```python
from build123d import *

# Parameters (mm, degrees)
SKETCH1_R           = 1.5
BOSS_EXTRUDE1_DEPTH = 2
SKETCH2_R           = 1.5
CUT_EXTRUDE1_DEPTH  = 55
FILLET1_R           = 1


with BuildPart() as part:
    # Sketch1 → Boss-Extrude1 (new body)
    with BuildSketch(Plane(origin=(0, 0, 0), x_dir=(1, 0, 0), z_dir=(0, 1, 0))):
        Polygon((0, 5), (0, -5), (3, -5), (3, 0), (8.68728571, 0), (8.68728571, -5), (11.68728571, -5), (11.68728571, 0), (38.51271429, 0), (38.51271429, -5), (41.51271429, -5), (41.51271429, 0), (47.2, 0), (47.2, -5), (50.2, -5), (50.2, 5), align=None)
        with Locations((2.5, 2.5)):
            Circle(SKETCH1_R, mode=Mode.SUBTRACT)
        with Locations((47.7, 2.5)):
            Circle(SKETCH1_R, mode=Mode.SUBTRACT)
    extrude(amount=BOSS_EXTRUDE1_DEPTH)

    # Sketch2 → Cut-Extrude1 (cut)
    with BuildSketch(Plane.ZY):
        with Locations((2.5, -0.5)):
            Circle(SKETCH2_R)
    extrude(amount=-CUT_EXTRUDE1_DEPTH, mode=Mode.SUBTRACT)

    # Fillet1
    fillet1_edges = [part.edges().sort_by_distance(p)[0] for p in [
        (50.2, 1, -5),
        (50.2, 1, 5),
        (38.51271429, 1, 5),
        (11.68728571, 1, 5),
        (0, 1, 5),
        (0, 1, -5),
    ]]
    fillet(fillet1_edges, radius=FILLET1_R)


solid = part.part
```
Work out the finished part from the listing and answer in its coordinate system (mm). A direction names the side the tool comes from. Round coordinates to 2 decimals unless told otherwise and drop trailing zeros. Loops run counter-clockwise (first coordinate to the right, second up) from the corner with the lowest first, then second, coordinate; pieces in that order, holes last. Notation, with made-up numbers: (-26.75, -20) -> (-9.75, -20) arc R19 cw to (-9.75, -13) -> close; hole circle Ø11 at (13.25, 3.25). An arc over 180 degrees is marked (long way). Write each question's results on one line, items separated by ' | '. Start each with the question number.
1. Section D-D (y = 0.35) is taken. State how many separate pieces and enclosed holes the cut face has, plus the area to 3 significant figures.
2. Given pin 1 Ø1.8 at (x, z) = (2.5, -2.5) entering from +Y; pin 2 Ø1 at (x, y) = (20, 1.5) entering from +Z, each flat-ended and moving along its own axis, determine where each tip first touches the part or whether it passes through.
3. Section A-A (x = 47.7) is taken. Determine the outline of the cut face in (y, z), plus the area to 3 significant figures.
4. A tool of negligible diameter and unlimited length cuts with its end or side. For faces 4 (the face through (25, 1, 0)), 5 (the face through (46.5, 1, -1.6)), from which of +Z, -Z, +X, -X, +Y, -Y can it reach the whole face along a straight path? Write none if from no direction.
5. Find the intervals of material crossed by probe 1 along X at (y, z) = (1.3, -2.5); probe 2 along X at (y, z) = (1.5, 2.5); probe 3 along X at (y, z) = (1.35, -1.75), in increasing order. Write a range as from..to.
6. For a pull along Z with two mould halves and no side action, classify faces 1 (the face through (8.687, 1.2, 2.5)), 2 (the face through (6, 1, 0)), 3 (the face through (48.7, 1, 2.5)) as +Z half, -Z half, draft (parallel to the pull), parting line (faces both ways), or undercut.
7. Section B-B (z = -2.5) is taken. Determine the outline of the cut face in (x, y).
8. Section C-C (z = 1.5) is taken. Determine the outline of the cut face in (x, y), plus the area to 3 significant figures.
Evaluation:
1) separate pieces: 5 | enclosed holes: 2 | area: 266 mm2
2) pin 1: passes through | pin 2: stops at z = 0
3) outline: (0, -5) -> (2, -5) -> (2, -4) -> (0, -4) -> close; (0, -1) -> (2, -1) -> (2, 5) -> (0, 5) -> (0, 3.91) arc R1.5 cw to (0, 1.09) -> close | area: 11.9 mm2
4) face 4: +Z, +Y, -Y | face 5: +Y, -Y
5) probe 1: x = 0..1, 4..46.2, 49.2..50.2 | probe 2: x = 0..3, 8.69..11.69, 38.51..41.51, 47.2..50.2 | probe 3: x = 0..1.2, 3.8..46.4, 49..50.2
6) face 1: draft | face 2: +Z half | face 3: undercut
7) outline: (0, 0) -> (1, 0) -> (1, 2) -> (0, 2) -> close; (4, 0) -> (46.2, 0) -> (46.2, 2) -> (4, 2) -> close; (49.2, 0) -> (50.2, 0) -> (50.2, 2) -> (49.2, 2) -> close
8) outline: (0, 0.62) -> (3, 0.62) -> (3, 2) -> (0, 2) -> close; (8.69, 0.62) -> (11.69, 0.62) -> (11.69, 2) -> (8.69, 2) -> close; (38.51, 0.62) -> (41.51, 0.62) -> (41.51, 2) -> (38.51, 2) -> close; (47.2, 0.62) -> (50.2, 0.62) -> (50.2, 2) -> (47.2, 2) -> close | area: 16.6 mm2
